from build123d import *

# Parameters (mm, degrees)
SKETCH_1_W               = 85
SKETCH_1_H               = 85
EXTRUDE_1_DEPTH          = 2
SKETCH_2_R               = 9
CUT_EXTRUDE_1_DEPTH      = 2
SKETCH_4_R               = 5
CUT_EXTRUDE_4_DEPTH      = 1
SKETCH_5_R               = 1
CUT_EXTRUDE_5_DEPTH      = 94.644624303
SKETCH_1_3_W             = 85
SKETCH_1_3_H             = 85
SKETCH_1_3_W_2           = 81
SKETCH_1_3_H_2           = 81
EXTRUDE_2_DEPTH          = 50
SKETCH_7_W               = 85
SKETCH_7_H               = 85
EXTRUDE_3_DEPTH          = 2
CUT_EXTRUDE_6_DEPTH      = 118.678046964
CUT_EXTRUDE_6_DEPTH_BACK = 118.678046964
CUT_EXTRUDE_7_DEPTH      = 122.55325139
CUT_EXTRUDE_7_DEPTH_BACK = 122.55325139
SKETCH_10_W              = 60.714285714
SKETCH_10_H              = 47.002651285
CHAMFER_4_SIZE           = 1
FILLET_1_R               = 2
FILLET_2_R               = 2
SKETCH_11_R              = 10
CUT_EXTRUDE_8_DEPTH      = 10
CUT_EXTRUDE_9_DEPTH      = 1


with BuildPart() as part:
    # 草图1 → 凸台-拉伸1 (new body)
    with BuildSketch(Plane.XY):
        with Locations((27.114602804, -20.102897196)):
            Rectangle(SKETCH_1_W, SKETCH_1_H)
    extrude(amount=EXTRUDE_1_DEPTH)

    # 草图2 → 切除-拉伸1 (cut)
    with BuildSketch(Plane(origin=(0, 0, 0), x_dir=(-1, 0, 0), z_dir=(0, 0, -1))):
        with Locations((-27.114602804, -20.102897196)):
            Circle(SKETCH_2_R)
    extrude(amount=-CUT_EXTRUDE_1_DEPTH, mode=Mode.SUBTRACT)

    # 草图4 → 切除-拉伸4 (cut)
    with BuildSketch(Plane(origin=(0, 0, 0), x_dir=(-1, 0, 0), z_dir=(0, 0, -1))):
        with Locations((-49.215493554, -42.995049302)):
            Circle(SKETCH_4_R)
        with Locations((-38.165048179, -31.548973249)):
            Circle(SKETCH_4_R)
        with Locations((-49.614602804, 2.397102804)):
            Circle(SKETCH_4_R)
        with Locations((-38.364602804, -8.852897196)):
            Circle(SKETCH_4_R)
        with Locations((-4.614602804, -42.602897196)):
            Circle(SKETCH_4_R)
        with Locations((-15.864602804, -31.352897196)):
            Circle(SKETCH_4_R)
        with Locations((-4.614602804, 2.397102804)):
            Circle(SKETCH_4_R)
        with Locations((-15.864602804, -8.852897196)):
            Circle(SKETCH_4_R)
    extrude(amount=-CUT_EXTRUDE_4_DEPTH, mode=Mode.SUBTRACT)

    # 草图5 → 切除-拉伸5 (cut, through all)
    with BuildSketch(Plane(origin=(0, 0, 0), x_dir=(-1, 0, 0), z_dir=(0, 0, -1))):
        with Locations((-4.614602804, -42.602897196)):
            Circle(SKETCH_5_R)
        with Locations((-15.864602804, -31.352897196)):
            Circle(SKETCH_5_R)
        with Locations((-15.864602804, -8.852897196)):
            Circle(SKETCH_5_R)
        with Locations((-4.614602804, 2.397102804)):
            Circle(SKETCH_5_R)
        with Locations((-38.364602804, -8.852897196)):
            Circle(SKETCH_5_R)
        with Locations((-49.614602804, 2.397102804)):
            Circle(SKETCH_5_R)
        with Locations((-49.215493554, -42.995049302)):
            Circle(SKETCH_5_R)
        with Locations((-38.165048179, -31.548973249)):
            Circle(SKETCH_5_R)
    extrude(amount=-CUT_EXTRUDE_5_DEPTH, mode=Mode.SUBTRACT)

    # 草图1<3> → 凸台-拉伸2 (add)
    with BuildSketch(Plane.XY):
        with Locations((27.114602804, -20.102897196)):
            Rectangle(SKETCH_1_3_W, SKETCH_1_3_H)
        with Locations((27.114602804, -20.102897196)):
            Rectangle(SKETCH_1_3_W_2, SKETCH_1_3_H_2, mode=Mode.SUBTRACT)
    extrude(amount=EXTRUDE_2_DEPTH)

    # 草图7 → 凸台-拉伸3 (add)
    with BuildSketch(Plane.XY.offset(50)):
        with Locations((27.114602804, -20.102897196)):
            Rectangle(SKETCH_7_W, SKETCH_7_H)
    extrude(amount=EXTRUDE_3_DEPTH)

    # 草图9 → 切除-拉伸6 (cut, two sides: drawn at the far end of the back side and taken through both)
    with BuildSketch(Plane(origin=(69.614602804, 0, 0), x_dir=(0, 0, -1), z_dir=(1, 0, 0)).offset(-CUT_EXTRUDE_6_DEPTH_BACK)):
        Polygon((-2.49772747, -50.460040053), (-49.5, -50.460040053), (-49.5, -38.482138921), (-2.49810108, -38.482138921), align=None)
        Polygon((-2.49848498, -26.174325768), (-49.5, -26.174325768), (-49.5, -14.031468625), (-2.498863735, -14.031468625), align=None)
        Polygon((-2.49924249, -1.888611482), (-49.5, -1.888611482), (-49.5, 10.254245661), (-2.499621245, 10.254245661), align=None)
    extrude(amount=CUT_EXTRUDE_6_DEPTH + CUT_EXTRUDE_6_DEPTH_BACK, mode=Mode.SUBTRACT)

    # 草图10 → 切除-拉伸7 (cut, two sides: drawn at the far end of the back side and taken through both)
    with BuildSketch(Plane.XZ.offset(62.602897196).offset(-CUT_EXTRUDE_7_DEPTH_BACK)):
        with Locations((27.114602804, 25.998674358)):
            Rectangle(SKETCH_10_W, SKETCH_10_H)
    extrude(amount=CUT_EXTRUDE_7_DEPTH + CUT_EXTRUDE_7_DEPTH_BACK, mode=Mode.SUBTRACT)

    # 倒角4
    chamfer_4_edges = [part.edges().sort_by_distance(p)[0] for p in [
        (36.114602804, -20.102897196, 0),
    ]]
    chamfer(chamfer_4_edges, length=CHAMFER_4_SIZE)

    # 圆角1
    fillet_1_edges = [part.edges().sort_by_distance(p)[0] for p in [
        (27.114602804, 22.397102804, 0),
        (69.614602804, -20.102897196, 0),
        (27.114602804, -62.602897196, 0),
        (-15.385397196, -20.102897196, 0),
    ]]
    fillet(fillet_1_edges, radius=FILLET_1_R)

    # 圆角2
    # the kernel refuses this fillet: 2 mm, written as the material it takes off along each edge
    with BuildSketch(Plane(origin=(-13.385397196, -60.602897196, 2), x_dir=(0, -1, 0), z_dir=(-1, 0, 0))) as fillet_2_piece_1_section:
        Polygon((0, 0), (FILLET_2_R, 0), (FILLET_2_R, -FILLET_2_R), (0, -FILLET_2_R), align=None)
    fillet_2_piece_1 = extrude(amount=FILLET_2_R, mode=Mode.PRIVATE)
    fillet_2_piece_1 = fillet_2_piece_1 - Plane(origin=(-13.385397196, -60.602897196, 2), x_dir=(0, 0.7071067811865475, 0.7071067811865475), z_dir=(-1, 0, 0)) * Sphere(FILLET_2_R, mode=Mode.PRIVATE)
    add(fillet_2_piece_1, mode=Mode.SUBTRACT)
    with BuildSketch(Plane(origin=(-15.385397196, -62.602897196, 2), x_dir=(0, 1, 0), z_dir=(0, 0, 1))) as fillet_2_piece_2:
        with BuildLine():
            CenterArc((FILLET_2_R, -FILLET_2_R), FILLET_2_R, 90, 90)
            Line((0, -FILLET_2_R), (0, 0))
            Line((0, 0), (FILLET_2_R, 0))
        make_face()
    extrude(amount=55, mode=Mode.SUBTRACT)

    # 草图11 → 切除-拉伸8 (cut)
    with BuildSketch(Plane.XY.offset(52)):
        with Locations((27.114602804, -19.602897196)):
            Circle(SKETCH_11_R)
    extrude(amount=-CUT_EXTRUDE_8_DEPTH, mode=Mode.SUBTRACT)

    # 草图12 → 切除-拉伸9 (cut)
    with BuildSketch(Plane.XY.offset(2)):
        Polygon((12.114602804, -20.102897196), (27.114602804, -35.102897196), (42.114602804, -20.102897196), (27.114602804, -5.102897196), align=None)
    extrude(amount=-CUT_EXTRUDE_9_DEPTH, mode=Mode.SUBTRACT)


solid = part.part
Could you check a few things on this model? Use its own coordinates, in mm. A direction names the side the tool comes from. Coordinates: 2 decimals unless noted, no trailing zeros. Loops run counter-clockwise (first coordinate to the right, second up) from the corner with the lowest first, then second, coordinate; pieces in that order, holes last.
1. For P1, Ø5, axis at x = 6, y = -41.5, coming from the -Z side; P2, Ø1.6, axis at x = 49.61, y = 2.4, coming from the -Z side; P3, Ø6, axis at y = -43, z = 6.5, coming from the +X side; P4, Ø2, axis at x = -14.5, y = 3, coming from the -Z side, each with a flat end and sliding along its axis, tell me the tip position at first contact or that it passes through.
2. I need wall thicknesses on L1, parallel to X at y = -58, z = 20; L2, parallel to Z at x = 44.5, y = -25; L3, parallel to Y at x = 65.5, z = 40.5. Which ranges of each line are inside material? Lowest first, please.
3. For faces 5 (the face through (-14, -45, 49.5)), 6 (the face through (57.472, 21, 26)), 7 (the face through (28.7, -62, 0.57)), 8 (the face through (35.48, -27.33, 0.49)), 9 (the face through (60, -60.603, 26)), which set-ups out of +Z, -Z, +X, -X, +Y, -Y let a thin tool reach every point of the face, with its end or its side?
4. Imagine slicing it at A-A (x = 2.5). Please give me the cut outline in (y, z), and give its area (3 significant figures).
5. Imagine slicing it at B-B (z = 9). Give the number of separate pieces and of enclosed holes in the cut face, and give its area (3 significant figures).
6. We'd pull the mould along Y, two halves only. Please class faces 1 (the face through (17, -29, 52)), 2 (the face through (69, 4, 49.5)), 3 (the face through (18, -11, 50)), 4 (the face through (27.71, 21.796, 0.57)): released by +Y, released by -Y, zero draft, split by the parting line, or undercut.
Computed values:
1. P1: stops at z = 1
1. P2: stops at z = 50
1. P3: passes through
1. P4: stops at z = 0
2. L1: x = -15.39 to -13.39, 67.61 to 69.61
2. L2: z = 0 to 2, 50 to 52
2. L3: y = -62.6 to -60.6, 20.4 to 22.4
3. face 5: +X, -X
3. face 6: +Y, -Y
3. face 7: -Z, +X, -X, -Y
3. face 8: -Z
3. face 9: none
4. outline: (-62.6, 2) arc R2 ccw to (-60.6, 0) - (-47.13, 0) - (-47.13, 1) - (-38.07, 1) - (-38.07, 0) - (-2.13, 0) - (-2.13, 1) - (6.93, 1) - (6.93, 0) - (20.4, 0) arc R2 ccw to (22.4, 2) - (22.4, 2.5) - (20.4, 2.5) - (20.4, 2) - (-60.6, 2) - (-60.6, 2.5) - (-62.6, 2.5) - close; (-62.6, 49.5) - (-60.6, 49.5) - (-60.6, 50) - (20.4, 50) - (20.4, 49.5) - (22.4, 49.5) - (22.4, 52) - (-62.6, 52) - close
4. area: 324 mm2
5. separate pieces: 8
5. enclosed holes: 0
5. area: 275 mm2
6. face 1: zero draft
6. face 2: undercut
6. face 3: undercut
6. face 4: released by +Y
